Can you work these out from the model? Positions are in its coordinate system, mm. Coordinates: 2 decimals unless noted, no trailing zeros. Order: outer loops, then holes, each group sorted by start corner. A loop starts at its lowest first (then second) coordinate and runs counter-clockwise, first axis right, second up.
```python
from build123d import *

# Parameters (mm, degrees)
SKETCH_1_W          = 10
SKETCH_1_H          = 5
EXTRUDE_1_DEPTH     = 65
SKETCH_2_R          = 1.675
CUT_EXTRUDE_1_DEPTH = 40
FILLET_1_R          = 5
SKETCH_3_W          = 36.824134977
SKETCH_3_H          = 78.201072097
CUT_EXTRUDE_2_DEPTH = 0.3


with BuildPart() as part:
    # 草图1 → 凸台-拉伸1 (new body)
    with BuildSketch(Plane.XY):
        with Locations((5, 2.5)):
            Rectangle(SKETCH_1_W, SKETCH_1_H)
    extrude(amount=EXTRUDE_1_DEPTH)

    # 草图2 → 切除-拉伸1 (cut)
    with BuildSketch(Plane(origin=(0, 5, 0), x_dir=(1, 0, 0), z_dir=(0, 1, 0))):
        with Locations(Location((5, -5, 0), (0, 0, 270))):
            Circle(SKETCH_2_R)
        with Locations(Location((5, -60, 0), (0, 0, 270))):
            Circle(SKETCH_2_R)
    extrude(amount=-CUT_EXTRUDE_1_DEPTH, mode=Mode.SUBTRACT)

    # 圆角1
    fillet_1_edges = [part.edges().sort_by_distance(p)[0] for p in [
        (0, 2.5, 65),
        (10, 2.5, 65),
        (0, 2.5, 0),
        (10, 2.5, 0),
    ]]
    fillet(fillet_1_edges, radius=FILLET_1_R - 0.0001)  # a hair under: the kernel refuses the full size

    # 草图3 → 切除-拉伸2 (cut)
    with BuildSketch(Plane(origin=(0, 5, 0), x_dir=(1, 0, 0), z_dir=(0, 1, 0))):
        with Locations((11.293579433, -34.071434458)):
            Rectangle(SKETCH_3_W, SKETCH_3_H)
    extrude(amount=-CUT_EXTRUDE_2_DEPTH, mode=Mode.SUBTRACT)


solid = part.part
```
1. Imagine slicing it at B-B on x = 9. Please give me the cut outline in (y, z).
Completed:
outline: (0, 2) - (4.7, 2) - (4.7, 63) - (0, 63) - close
2. Please list where these lines run through material, in increasing order: probe 1 along X at (y, z) = (2, 60) (3 decimals); probe 2 along Z at (x, y) = (6, 1.7); probe 3 along X at (y, z) = (2.55, 6).
Completed:
probe 1: x = 0 to 3.325, 6.675 to 10
probe 2: z = 0.1 to 3.66, 6.34 to 58.66, 61.34 to 64.9
probe 3: x = 0 to 3.66, 6.34 to 10
3. Thinking about a two-plate mould opening in X: for faces 1 (the cylindrical face through (3.514, 2.383, 5.773)), 2 (the cylindrical face through (1, 2, 63)), 3 (the flat face through (10, 2, 32)), which applies, pulls with the +X half, pulls with the -X half, needs draft (parallel to the pull), parting line crosses it, or undercut?
Completed:
face 1: undercut
face 2: pulls with the -X half
face 3: pulls with the +X half
4. Imagine slicing it at A-A on y = 3.9. Give the number of separate pieces and of enclosed holes in the cut face, then the cut area to 3 significant figures.
Completed:
separate pieces: 1
enclosed holes: 2
area: 611 mm2
